Model file for the job. Use its own axes, mm. Face numbers are marked on the shaded views. A direction names the side the tool comes from. Give positions to 0.01 mm unless a question says otherwise; leave off trailing zeros. Loops run counter-clockwise (first coordinate to the right, second up) from the corner with the lowest first, then second, coordinate; pieces in that order, holes last. Notation, with made-up numbers: M 41.5,66.25 L 54.5,66.25 A25 ccw 54.5,87.25 Z; hole C 69,25.25 d2. An arc over 180 degrees is marked long. Answer in a Markdown table with one row per item.
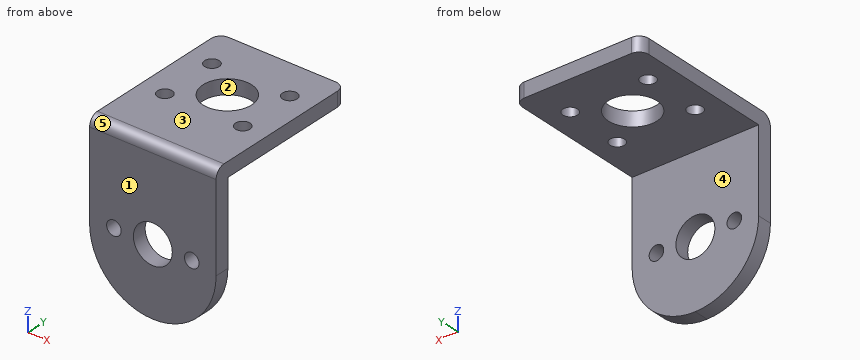
```python
from build123d import *

# Parameters (mm, degrees)
SKETCH1_W           = 26
SKETCH1_H           = 33
SKETCH1_R           = 5
SKETCH1_R_2         = 1.5
BOSS_EXTRUDE1_DEPTH = 3
SKETCH2_W           = 26
SKETCH2_H           = 3
BOSS_EXTRUDE2_DEPTH = 30
SKETCH3_R           = 4
SKETCH3_R_2         = 1.5
CUT_EXTRUDE1_DEPTH  = 4
FILLET1_R           = 2
FILLET2_R           = 2


with BuildPart() as part:
    # Sketch1 → Boss-Extrude1 (new body)
    with BuildSketch(Plane.XY):
        Rectangle(SKETCH1_W, SKETCH1_H)
        with Locations((0, 2.5)):
            Circle(SKETCH1_R, mode=Mode.SUBTRACT)
        with Locations((-8, 8.5)):
            Circle(SKETCH1_R_2, mode=Mode.SUBTRACT)
        with Locations((8, 8.5)):
            Circle(SKETCH1_R_2, mode=Mode.SUBTRACT)
        with Locations((8, -3.5)):
            Circle(SKETCH1_R_2, mode=Mode.SUBTRACT)
        with Locations((-8, -3.5)):
            Circle(SKETCH1_R_2, mode=Mode.SUBTRACT)
    extrude(amount=BOSS_EXTRUDE1_DEPTH)

    # Sketch2 → Boss-Extrude2 (add)
    with BuildSketch(Plane(origin=(0, 0, 0), x_dir=(-1, 0, 0), z_dir=(0, 0, -1))):
        with Locations((0, -15)):
            Rectangle(SKETCH2_W, SKETCH2_H)
    extrude(amount=BOSS_EXTRUDE2_DEPTH)

    # Sketch3 → Cut-Extrude1 (cut, through all)
    with BuildSketch(Plane(origin=(0, -13.5, 0), x_dir=(1, 0, 0), z_dir=(0, 1, 0))):
        with BuildLine():
            Line((0, 30), (-13, 30))
            Line((-13, 30), (-13, 17))
            ThreePointArc((-13, 17), (-9.192388155, 26.192388155), (0, 30))
        make_face()
        with BuildLine():
            Line((13, 30), (0, 30))
            ThreePointArc((0, 30), (9.192388162, 26.192388149), (13, 16.999999981))
            Line((13, 16.999999981), (13, 30))
        make_face()
        with Locations((0, 16)):
            Circle(SKETCH3_R)
        with Locations((-8, 16)):
            Circle(SKETCH3_R_2)
        with Locations((8, 16)):
            Circle(SKETCH3_R_2)
    extrude(amount=-CUT_EXTRUDE1_DEPTH, mode=Mode.SUBTRACT)

    # Fillet1
    fillet1_edges = [part.edges().sort_by_distance(p)[0] for p in [
        (-13, 16.5, 1.5),
        (13, 16.5, 1.5),
    ]]
    fillet(fillet1_edges, radius=FILLET1_R)

    # Fillet2
    fillet2_edges = [part.edges().sort_by_distance(p)[0] for p in [
        (0, -16.5, 3),
    ]]
    fillet(fillet2_edges, radius=FILLET2_R)


solid = part.part
```
(1) Wall check: L1, parallel to X at y = -15, z = -16; L2, parallel to Y at x = -8, z = 2.2; L3, parallel to Z at x = 10, y = -6.5. Give the ranges that are in metal, low to high.
Established:
| item | result |
|---|---|
| L1 | x = -13 to -9.5, -6.5 to -4, 4 to 6.5, 9.5 to 13 |
| L2 | y = -16.1 to -5, -2 to 7, 10 to 16.5 |
| L3 | z = 0 to 3 |
(2) Saw through at B-B, the plane y = -3.5. Give the cut face in (x, z), and give its area (3 significant figures).
Established:
| item | result |
|---|---|
| outline | M -13,0 L -9.5,0 L -9.5,3 L -13,3 Z; M -6.5,0 L 6.5,0 L 6.5,3 L -6.5,3 Z; M 9.5,0 L 13,0 L 13,3 L 9.5,3 Z |
| area | 60.0 mm2 |
(3) Flat gauge pins, fed straight in: P1, Ø6, axis at x = -4.5, y = 6.5, coming from the -Z side; P2, Ø10, axis at x = -2, z = -18.5, coming from the +Y side; P3, Ø3, axis at y = -12.5, z = -6.5, coming from the -X side. Where does each tip first touch, or does it go through?
Established:
| item | result |
|---|---|
| P1 | stops at z = 0 |
| P2 | stops at y = -13.5 |
| P3 | stops at x = -13 |
(4) Saw through at A-A, the plane z = -16. Give the cut face in (x, y).
Established:
| item | result |
|---|---|
| outline | M -13,-16.5 L -9.5,-16.5 L -9.5,-13.5 L -13,-13.5 Z; M -6.5,-16.5 L -4,-16.5 L -4,-13.5 L -6.5,-13.5 Z; M 4,-16.5 L 6.5,-16.5 L 6.5,-13.5 L 4,-13.5 Z; M 9.5,-16.5 L 13,-16.5 L 13,-13.5 L 9.5,-13.5 Z |
(5) Saw through at D-D, the plane y = 2.5. Give the cut face in (x, z).
Established:
| item | result |
|---|---|
| outline | M -13,0 L -5,0 L -5,3 L -13,3 Z; M 5,0 L 13,0 L 13,3 L 5,3 Z |
(6) Saw through at C-C, the plane x = -8. Give the cut face in (y, z), and give its area (3 significant figures).
Established:
| item | result |
|---|---|
| outline | M -16.5,-27.25 L -13.5,-27.25 L -13.5,-17.5 L -16.5,-17.5 Z; M -16.5,-14.5 L -13.5,-14.5 L -13.5,0 L -5,0 L -5,3 L -14.5,3 A2 ccw -16.5,1 Z; M -2,0 L 7,0 L 7,3 L -2,3 Z; M 10,0 L 16.5,0 L 16.5,3 L 10,3 Z |
| area | 153 mm2 |
(7) Which spindle directions (+Z, -Z, +X, -X, +Y, -Y) get a long thin tool onto all of the face, cutting with end or side? Do the marked faces 4 and 5. Say none if no direction does.
Established:
| item | result |
|---|---|
| face 4 | -Z, +X, -X, +Y |
| face 5 | +Z, +X, -X, -Y |
(8) Mould opens along Y. For the marked faces 1, 2 and 3 say: pulls with the +Y half, pulls with the -Y half, needs draft (parallel to the pull), parting line crosses it, or undercut.
Established:
| item | result |
|---|---|
| face 1 | pulls with the -Y half |
| face 2 | undercut |
| face 3 | needs draft |
